Input: part model. Units: mm. Frame: model coordinates. Give positions to 0.01 mm unless a question says otherwise; leave off trailing zeros. Loops run counter-clockwise (first coordinate to the right, second up) from the corner with the lowest first, then second, coordinate; pieces in that order, holes last. Notation, with made-up numbers: M 47.25,-35.5 L 90.25,-35.5 A17 cw 90.25,-15.5 Z; hole C -24.5,-38 d2. An arc over 180 degrees is marked long. One line per item, written item: value. Start each with the question number.
(1) Section C-C on y = 54.5. Output: boundary loops of the cut face in (x, z).
(2) Ray query, line 1 along Y through (x, z) = (3.85, -142.24) (3 decimals); line 2 along Y through (x, z) = (0.5, 23); line 3 along Y through (x, z) = (4.6, -140). Return the intervals inside material, ascending. Write a range as from..to.
(3) Section A-A on z = -5. Output: boundary loops of the cut face in (x, y).
(4) Section B-B on x = 3.65. Output: boundary loops of the cut face in (y, z) (3 decimals).
(5) Pin query (flat end, axial travel): P1, Ø5.5, axis at y = -147.65, z = 28.7, coming from the +X side; P2, Ø2.5, axis at x = 2.5, y = 122.5, coming from the +Z side; P3, Ø2.5, axis at x = 3.5, y = -132, coming from the +Z side. Return the tip coordinate at first contact, or that it passes through.
(6) Section D-D on z = -84. Output: boundary loops of the cut face in (x, y), plus the area to 3 significant figures.
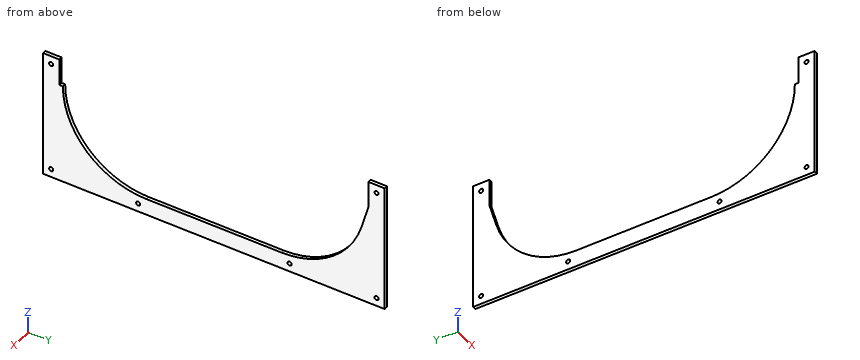
```python
from build123d import *

# Parameters (mm, degrees)
SKETCH1_R           = 3.175
BOSS_EXTRUDE3_DEPTH = 5.4102
CUT_EXTRUDE1_DEPTH  = 5.4102


with BuildPart() as part:
    # Sketch1 → Boss-Extrude3 (new body)
    with BuildSketch(Plane(origin=(0, 0, 0), x_dir=(0, 0, -1), z_dir=(1, 0, 0))):
        with BuildLine():
            ThreePointArc((129.54, 0), (124.431830765, -36.01848265), (109.510185389, -69.196321406))
            ThreePointArc((109.510185389, -69.196321406), (62.517678, -113.455504659), (0, -129.54))
            Line((0, -129.54), (0, -134.9502))
            Line((0, -134.9502), (-41.402, -134.9502))
            Line((-41.402, -134.9502), (-41.402, -160.3502))
            Line((-41.402, -160.3502), (154.94, -160.3502))
            Line((154.94, -160.3502), (154.94, 369.88496))
            Line((154.94, 369.88496), (-41.402, 369.88496))
            Line((-41.402, 369.88496), (-41.402, 344.48496))
            Line((-41.402, 344.48496), (0, 344.48496))
            Line((0, 344.48496), (0, 339.07476))
            ThreePointArc((0, 339.07476), (62.517678, 322.990264659), (109.510185389, 278.731081406))
            ThreePointArc((109.510185389, 278.731081406), (124.431830765, 245.55324265), (129.54, 209.53476))
            Line((129.54, 209.53476), (129.54, 0))
        make_face()
        with Locations((-28.702, -147.6502)):
            Circle(SKETCH1_R, mode=Mode.SUBTRACT)
        with Locations((142.24, -147.6502)):
            Circle(SKETCH1_R, mode=Mode.SUBTRACT)
        with Locations((142.24, -12.7)):
            Circle(SKETCH1_R, mode=Mode.SUBTRACT)
        with Locations((-28.702, 357.18496)):
            Circle(SKETCH1_R, mode=Mode.SUBTRACT)
        with Locations((142.24, 222.23476)):
            Circle(SKETCH1_R, mode=Mode.SUBTRACT)
        with Locations((142.24, 357.18496)):
            Circle(SKETCH1_R, mode=Mode.SUBTRACT)
    extrude(amount=BOSS_EXTRUDE3_DEPTH)

    # Sketch2 → Cut-Extrude1 (cut)
    with BuildSketch(Plane(origin=(5.4102, 0, 0), x_dir=(0, 0, -1), z_dir=(1, 0, 0))):
        Polygon((0, 344.48496), (36.311280568, 333.881462825), (0, 339.07476), align=None)
    extrude(amount=-CUT_EXTRUDE1_DEPTH, mode=Mode.SUBTRACT)


solid = part.part
```
Output values:
1. outline: M 0,-154.94 L 5.41,-154.94 L 5.41,-129.54 L 0,-129.54 Z
2. line 1: y = -160.35..-150.825, -144.475..-15.875, -9.525..219.06, 225.41..354.01, 360.36..369.885
2. line 2: y = -160.35..-134.95, 344.48..369.88
2. line 3: y = -160.35..-149.9, -145.4..-14.95, -10.45..219.98, 224.48..354.93, 359.44..369.88
3. outline: M 0,-160.35 L 5.41,-160.35 L 5.41,-129.44 L 0,-129.44 Z; M 0,343.02 L 5.41,343.02 L 5.41,369.88 L 0,369.88 Z
4. outline: M -160.35,-154.94 L 369.885,-154.94 L 369.885,41.402 L 344.485,41.402 L 344.485,0 L 333.881,-36.311 A129.54 cw 209.535,-129.54 L 0,-129.54 A129.54 cw -129.54,0 L -134.95,0 L -134.95,41.402 L -160.35,41.402 Z; hole C -147.65,-142.24 d6.35; hole C -147.65,28.702 d6.35; hole C -12.7,-142.24 d6.35; hole C 222.235,-142.24 d6.35; hole C 357.185,-142.24 d6.35; hole C 357.185,28.702 d6.35
5. P1: passes through
5. P2: stops at z = -129.54
5. P3: stops at z = 0
6. outline: M 0,-160.35 L 5.41,-160.35 L 5.41,-98.61 L 0,-98.61 Z; M 0,308.15 L 5.41,308.15 L 5.41,369.88 L 0,369.88 Z
6. area: 668 mm²
